Job drawing, mm, ordinate dimensions from the low corner. One solid piece. A direction names the side the tool comes from. Coordinates: 2 decimals unless noted, no trailing zeros. Loops run counter-clockwise (first coordinate to the right, second up) from the corner with the lowest first, then second, coordinate; pieces in that order, holes last. Notation, with made-up numbers: (21, 39) - (50, 39) arc R27 cw to (50, 67) - close; hole circle Ø3 at (10, 69). An arc over 180 degrees is marked (long way). Use a Markdown table: item, result. Add a question column.
1. Pull direction Y, two halves, no side cores. Call the marked faces 1, 2, 3 and 4: pulls with the +Y half, pulls with the -Y half, needs draft (parallel to the pull), parting line crosses it, or undercut.
2. Band-saw the part on C-C, the plane x = 18. Give the cut face in (y, z), plus the area to 3 significant figures.
3. Band-saw the part on A-A, the plane y = 2. Give the cut face in (x, z), plus the area to 3 significant figures.
4. Drop flat-ended pins along their axis: pin 1 (5 mm diameter, centred on x = 20, y = 7.5, fed in from +Z); pin 2 (2 mm diameter, centred on x = 21.5, y = 11.5, fed in from +Z); pin 3 (5 mm diameter, centred on x = 14.5, y = 11, fed in from -Z). Give the stop position or say it passes through.
5. Band-saw the part on D-D, the plane x = 8. Give the cut face in (y, z), plus the area to 3 significant figures.
6. Wall check: probe 1 along Z at (x, y) = (18, 10); probe 2 along Z at (x, y) = (29.5, 6); probe 3 along Y at (x, z) = (8.5, 4). Give the ranges that are in metal, low to high. Write a range as [from, to].
7. 3-axis set-ups, long thin cutter, end or side, ignore diameter. For the marked faces 5, 6 and 7: which of +Z, -Z, +X, -X, +Y, -Y reach the whole face in a straight line?
8. Band-saw the part on B-B, the plane z = 14.25. Give the cut face in (x, y).
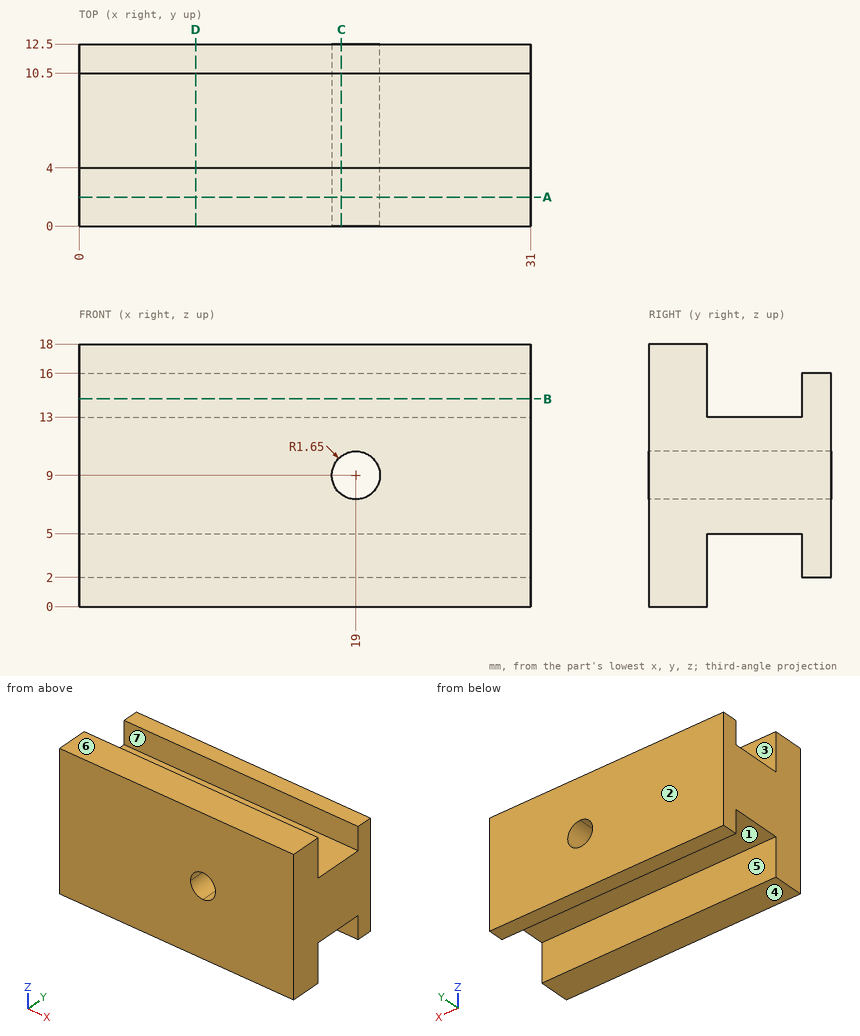
Geometry check:
| question | item | result |
|---|---|---|
| 1 | face 1 | undercut |
| 1 | face 2 | pulls with the +Y half |
| 1 | face 3 | undercut |
| 1 | face 4 | needs draft |
| 2 | outline | (0, 0) - (4, 0) - (4, 5) - (10.5, 5) - (10.5, 2) - (12.5, 2) - (12.5, 7.69) - (0, 7.69) - close; (0, 10.31) - (12.5, 10.31) - (12.5, 16) - (10.5, 16) - (10.5, 13) - (4, 13) - (4, 18) - (0, 18) - close |
| 2 | area | 119 mm^2 |
| 3 | outline | (0, 0) - (31, 0) - (31, 18) - (0, 18) - close; hole circle Ø3.3 at (19, 9) |
| 3 | area | 549 mm^2 |
| 4 | pin 1 | stops at z = 13 |
| 4 | pin 2 | stops at z = 16 |
| 4 | pin 3 | stops at z = 2 |
| 5 | outline | (0, 0) - (4, 0) - (4, 5) - (10.5, 5) - (10.5, 2) - (12.5, 2) - (12.5, 16) - (10.5, 16) - (10.5, 13) - (4, 13) - (4, 18) - (0, 18) - close |
| 5 | area | 152 mm^2 |
| 6 | probe 1 | z = [5, 7.69], [10.31, 13] |
| 6 | probe 2 | z = [5, 13] |
| 6 | probe 3 | y = [0, 4], [10.5, 12.5] |
| 7 | face 5 | -Z, +X, -X |
| 7 | face 6 | +Z, +X, -X, +Y, -Y |
| 7 | face 7 | +Z, +X, -X |
| 8 | outline | (0, 0) - (31, 0) - (31, 4) - (0, 4) - close; (0, 10.5) - (31, 10.5) - (31, 12.5) - (0, 12.5) - close |
